The listing builds one solid part. Answer for the finished solid, in the listing's coordinates (mm). A direction names the side the tool comes from. Round coordinates to 2 decimals unless told otherwise and drop trailing zeros. Order: outer loops, then holes, each group sorted by start corner. A loop starts at its lowest first (then second) coordinate and runs counter-clockwise, first axis right, second up. Notation, with made-up numbers: (17.5, 51.25) - (58.5, 51.25) arc R32 ccw to (58.5, 81.25) - close; hole circle Ø3 at (57.25, 36.25). An arc over 180 degrees is marked (long way). One line per item, written item: value. Start each with the question number.
1. Section B-B, the plane y = -3.75 is taken. Give the vertices of the cut face in (x, z), then the cut area to 3 significant figures.
2. Section C-C, the plane z = 0 is taken. Give the vertices of the cut face in (x, y).
3. Straight lines are drawn through the part: line 1 (Z direction, x = 0, y = 2.5); line 2 (X direction, y = -3.75, z = 22); line 3 (X direction, y = -4, z = 13). For each, find the intervals that lie inside material, in ascending order.
4. Section D-D, the plane x = 9 is taken. Give the vertices of the cut face in (y, z), then the cut area to 3 significant figures.
5. Flat-ended cylindrical pins translate along their axes: P1, Ø3, axis at y = 3.5, z = 17, coming from the +X side; P2, Ø1, axis at y = -2.5, z = 20, coming from the +X side; P3, Ø1.3, axis at y = -3.5, z = 17.5, coming from the -X side. Find the tip coordinate at first contact, or state that the pin passes through.
6. Section A-A, the plane x = 0 is taken. Give the vertices of the cut face in (y, z), then the cut area to 3 significant figures.
7. A tool of negligible diameter and unlimited length cuts with its end or side. For faces 1 (the flat face through (0, 0, 6)), 2 (the flat face through (1.15, -4, 18)), 3 (the flat face through (2, 5, 17)), from which of +Z, -Z, +X, -X, +Y, -Y can it reach the whole face along a straight path? Write none if from no direction.
8. For a pull along X with two mould halves and no side action, classify faces 4 (the flat face through (1.15, 4, 18)), 5 (the flat face through (10, 0, 26)), 6 (the flat face through (-7.477, -0.07, 10.62)), 7 (the cylindrical face through (-0.54, 0.07, -2.44)) as released by +X, released by -X, zero draft, split by the parting line, or undercut.
from build123d import *

# Parameters (mm, degrees)
F0_R     = 2.5
F1_DEPTH = 5
F2_W     = 2.3
F2_H     = 10
F3_DEPTH = 24
F5_W     = 10
F5_H     = 5
F7_W     = 13
F7_H     = 6


with BuildPart() as f1:
    # F0 (on Front) → F1 (new body, symmetric)
    with BuildSketch(Plane.XZ):
        with BuildLine():
            ThreePointArc((-4.881421, -1.082464), (0, -5), (4.881421, -1.082464))
            Line((4.881421, -1.082464), (10, 22))
            Line((10, 22), (10, 30))
            Line((10, 30), (-10, 30))
            Line((-10, 30), (-10, 22))
            Line((-10, 22), (-4.881421, -1.082464))
        make_face()
        Circle(F0_R, mode=Mode.SUBTRACT)
    extrude(amount=F1_DEPTH, both=True)

    # F2 (on face) → F3 (cut)
    with BuildSketch(Plane.XY.offset(30)):
        Rectangle(F2_W, F2_H)
    extrude(amount=-F3_DEPTH, mode=Mode.SUBTRACT)

    # F5 (on offset) → F8 section 0
    with BuildSketch(Plane.XY.offset(6)):
        Rectangle(F5_W, F5_H)
    # F7 (on offset) → F8 section 1
    with BuildSketch(Plane.XY.offset(30)):
        Rectangle(F7_W, F7_H)
    loft(mode=Mode.SUBTRACT)


solid = f1.part
Answer list:
1. outline: (-10, 22) - (-4.88, -1.08) arc R5 ccw to (4.88, -1.08) - (10, 22) - (10, 30) - (1.15, 30) - (1.15, 6) - (-1.15, 6) - (-1.15, 30) - (-10, 30) - close; hole circle Ø5 at (0, 0)
1. area: 457 mm²
2. outline: (-5.12, -5) - (-2.5, -5) - (-2.5, 5) - (-5.12, 5) - close; (2.5, -5) - (5.12, -5) - (5.12, 5) - (2.5, 5) - close
3. line 1: z = -5 to -2.5, 2.5 to 6
3. line 2: x = -10 to -1.15, 1.15 to 10
3. line 3: x = -8 to -1.15, 1.15 to 8
4. outline: (-5, 17.49) - (5, 17.49) - (5, 30) - (-5, 30) - close
4. area: 125 mm²
5. P1: stops at x = 9.22
5. P2: stops at x = 9.67
5. P3: stops at x = -9.15
6. outline: (-5, -5) - (5, -5) - (5, -2.5) - (-5, -2.5) - close; (-5, 2.5) - (5, 2.5) - (5, 6) - (-5, 6) - close
6. area: 60.0 mm²
7. face 1: +Z
7. face 2: +Z, +Y, -Y
7. face 3: +Z, -Z, +X, -X, +Y
8. face 4: undercut
8. face 5: released by +X
8. face 6: released by -X
8. face 7: undercut
